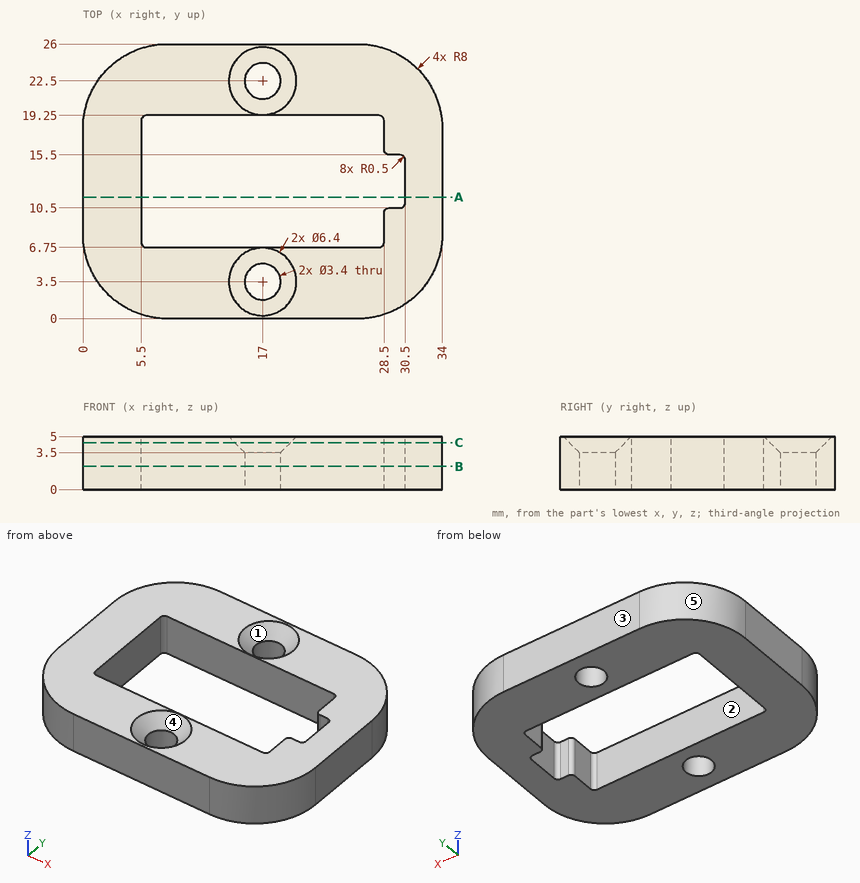
Verification items for this drawing (mm, ordinates from the low corner). A direction names the side the tool comes from. Coordinates: 2 decimals unless noted, no trailing zeros. Write each loop counter-clockwise with the first axis right and the second up, starting at its lowest first coordinate (ties: lowest second). Pieces come first, ordered by that corner, then holes. Notation, with made-up numbers: M -6.75,-15.5 L 19.25,-15.5 A21 cw 19.25,18.5 Z; hole C -18.75,42.25 d4. An arc over 180 degrees is marked long. Answer as a JSON object with one key per item and string values. Group by question number.
(1) Cross-section at A-A, the plane y = 11.5. Record the cut outline in (x, z), and give its area (3 significant figures).
(2) Gauge pin test, flat ends, axial feed: pin 1 (1.1 mm diameter, centred on x = 29.5, z = 2.5, fed in from +Y); pin 2 (4.5 mm diameter, centred on x = 17, y = 22.5, fed in from +Z); pin 3 (0.8 mm diameter, centred on x = 29.5, z = 2, fed in from -Y) (3 decimals). Record the tip position at first contact, or that the pin passes through.
(3) Tool access check on the marked faces 1 and 2. Record the directions out of +Z, -Z, +X, -X, +Y, -Y that give a thin tool (end or side, any length) a straight path to the whole face; none if there is none.
(4) Cross-section at C-C, the plane z = 4.45. Record the cut outline in (x, y).
(5) Cross-section at B-B, the plane z = 2.2. Record the cut outline in (x, y), and give its area (3 significant figures).
(6) Release check for a two-part mould opening along X. For the marked faces 3, 4 and 5 record: +X half, -X half, draft (parallel to the pull), parting line (faces both ways), or undercut.
(7) Material ranges on line 1 (Y direction, x = 25, z = 0.75); line 2 (X direction, y = 14.5, z = 1.4); line 3 (X direction, y = 9.5, z = 1.65), recorded low to high.
Reply:
{
 "1": {"outline": "M 0,0 L 5.5,0 L 5.5,5 L 0,5 Z; M 30.5,0 L 34,0 L 34,5 L 30.5,5 Z", "area": "45.0 mm²"},
 "2": {"pin 1": "y = 25.44", "pin 2": "z = 4.05", "pin 3": "y = 0.625"},
 "3": {"face 1": "+Z", "face 2": "+Z, -Z"},
 "4": {"outline": "M 0,8 A8 ccw 8,0 L 26,0 A8 ccw 34,8 L 34,18 A8 ccw 26,26 L 8,26 A8 ccw 0,18 Z; hole M 5.5,7.25 A0.5 ccw 6,6.75 L 28,6.75 A0.5 ccw 28.5,7.25 L 28.5,10 A0.5 cw 29,10.5 L 30,10.5 A0.5 ccw 30.5,11 L 30.5,15 A0.5 ccw 30,15.5 L 29,15.5 A0.5 cw 28.5,16 L 28.5,18.75 A0.5 ccw 28,19.25 L 6,19.25 A0.5 ccw 5.5,18.75 Z; hole C 17,3.5 d5.3; hole C 17,22.5 d5.3"},
 "5": {"outline": "M 0,8 A8 ccw 8,0 L 26,0 A8 ccw 34,8 L 34,18 A8 ccw 26,26 L 8,26 A8 ccw 0,18 Z; hole M 5.5,7.25 A0.5 ccw 6,6.75 L 28,6.75 A0.5 ccw 28.5,7.25 L 28.5,10 A0.5 cw 29,10.5 L 30,10.5 A0.5 ccw 30.5,11 L 30.5,15 A0.5 ccw 30,15.5 L 29,15.5 A0.5 cw 28.5,16 L 28.5,18.75 A0.5 ccw 28,19.25 L 6,19.25 A0.5 ccw 5.5,18.75 Z; hole C 17,3.5 d3.4; hole C 17,22.5 d3.4", "area": "514 mm²"},
 "6": {"face 3": "draft", "face 4": "undercut", "face 5": "-X half"},
 "7": {"line 1": "0 to 6.75, 19.25 to 26", "line 2": "0 to 5.5, 30.5 to 34", "line 3": "0 to 5.5, 28.5 to 34"}
}
